```python
from build123d import *

# Parameters (mm, degrees)
F0_W     = 200
F0_H     = 50
F0_R     = 20
F1_DEPTH = 20
F2_R     = 24.99999


# Not quite as in the source:
# - a fillet or chamfer is up to 0.001 mm smaller than in the source, because OpenCascade refuses the exact size


with BuildPart() as f1:
    # F0 (on Top) → F1 (new body)
    with BuildSketch(Plane.XY):
        with Locations((100, 25)):
            Rectangle(F0_W, F0_H)
        with Locations((100, 25)):
            Circle(F0_R, mode=Mode.SUBTRACT)
    extrude(amount=F1_DEPTH)

    # F2 (radius 25 in the source; OpenCascade refuses exactly that, so slightly less here)
    f2_edges = [f1.edges().sort_by_distance(p)[0] for p in [
        (200, 0, 10),
        (0, 50, 10),
        (0, 0, 10),
        (200, 50, 10),
    ]]
    fillet(f2_edges, radius=F2_R)


solid = f1.part
```
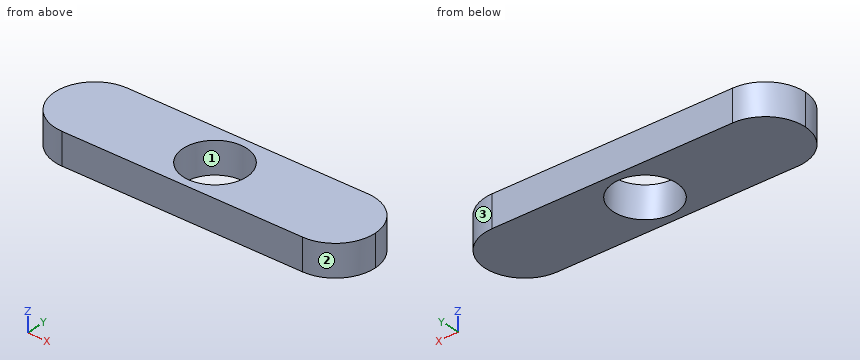
Geometry check sheet. Reference: the model listing, model coordinates, mm. Face numbers are marked on the shaded views. Round coordinates to 2 decimals unless told otherwise and drop trailing zeros. Order: outer loops, then holes, each group sorted by start corner. A loop starts at its lowest first (then second) coordinate and runs counter-clockwise, first axis right, second up. Notation, with made-up numbers: (-31.75, 87) - (5.25, 87) arc R10 ccw to (5.25, 103) - close; hole circle Ø2 at (46, 64.5). An arc over 180 degrees is marked (long way). Use a Markdown table: item, result. Add a question column.
1) Mould release check, pull along Y, two halves, no side actions. Record for the marked faces 1, 2 and 3: released by +Y, released by -Y, zero draft, split by the parting line, or undercut.
2) Thickness scan on line 1 along Y through (x, z) = (100, 15.5); line 2 along X through (y, z) = (26, 16.25); line 3 along X through (y, z) = (39, 2.5). Record the ranges inside material, lowest first.
3) Gauge pin test, flat ends, axial feed: P1, Ø2, axis at y = 7.5, z = 13, coming from the -X side; P2, Ø1.5, axis at y = 5.5, z = 9.5, coming from the +X side. Record the tip position at first contact, or that the pin passes through.
4) Section check B-B (x = 100). Record the cut outline in (y, z).
5) Section check C-C (y = 27.5). Record the cut outline in (x, z).
Established:
| question | item | result |
|---|---|---|
| 1 | face 1 | undercut |
| 1 | face 2 | released by -Y |
| 1 | face 3 | released by +Y |
| 2 | line 1 | 0 to 5, 45 to 50 |
| 2 | line 2 | 0.02 to 80.03, 119.97 to 199.98 |
| 2 | line 3 | 4.29 to 85.72, 114.28 to 195.71 |
| 3 | P1 | x = 6.22 |
| 3 | P2 | x = 191.54 |
| 4 | outline | (0, 0) - (5, 0) - (5, 20) - (0, 20) - close; (45, 0) - (50, 0) - (50, 20) - (45, 20) - close |
| 5 | outline | (0.13, 0) - (80.16, 0) - (80.16, 20) - (0.13, 20) - close; (119.84, 0) - (199.87, 0) - (199.87, 20) - (119.84, 20) - close |
